Input: part model. Units: mm. Frame: model coordinates. Give positions to 0.01 mm unless a question says otherwise; leave off trailing zeros. Write each loop counter-clockwise with the first axis right and the second up, starting at its lowest first coordinate (ties: lowest second). Pieces come first, ordered by that corner, then holes. Notation, with made-up numbers: (-19.75, 66) - (-10.75, 66) arc R19 ccw to (-10.75, 90) - close; hole circle Ø7 at (-7.75, 45). An arc over 180 degrees is marked (long way). Use a Markdown table: item, result. Add a question column.
1. Section query A-A, the plane x = 113.5. Return loops of the section in (y, z).
2. Material intervals for probe 1 along Z at (x, y) = (45, -2.15); probe 2 along X at (y, z) = (-1.7, -7.5); probe 3 along X at (y, z) = (-0.35, 34), sorted ascending.
3. Section query B-B, the plane z = 38. Return loops of the section in (x, y), plus the area to 3 significant figures.
4. Pin query (flat end, axial travel): pin 1 (1.5 mm diameter, centred on x = 30.5, y = -1.5, fed in from -Z). Return the tip coordinate at first contact, or that it passes through.
5. Section query D-D, the plane z = -25. Return loops of the section in (x, y), plus the area to 3 significant figures.
6. Section query C-C, the plane y = -1.55. Count the separate pieces of the cut face and the enclosed holes in it, plus the area to 3 significant figures.
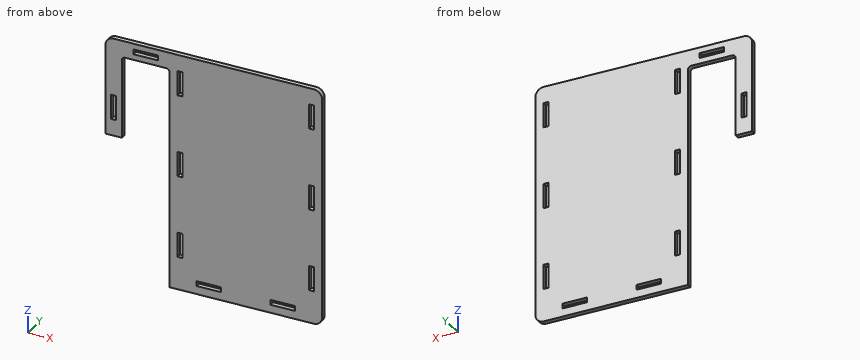
```python
from build123d import *

# Parameters (mm, degrees)
F1_W     = 15
F1_H     = 3
F1_W_2   = 3
F1_H_2   = 15
F2_DEPTH = 3


with BuildPart() as f2:
    # F1 (on Front) → F2 (new body)
    with BuildSketch(Plane.XZ):
        with BuildLine():
            Line((0, 55), (0, 0))
            Line((0, 0), (10, 0))
            Line((10, 0), (10, 48))
            ThreePointArc((10, 48), (10.5857864376, 49.4142135624), (12, 50))
            Line((12, 50), (37, 50))
            ThreePointArc((37, 50), (38.4142135624, 49.4142135624), (39, 48))
            Line((39, 48), (39, -85))
            Line((39, -85), (127, -85))
            ThreePointArc((127, -85), (130.5355339059, -83.5355339059), (132, -80))
            Line((132, -80), (132, 55))
            ThreePointArc((132, 55), (130.5355339059, 58.5355339059), (127, 60))
            Line((127, 60), (5, 60))
            ThreePointArc((5, 60), (1.4644660941, 58.5355339059), (0, 55))
        make_face()
        with Locations((63, -78.5)):
            Rectangle(F1_W, F1_H, mode=Mode.SUBTRACT)
        with Locations((45.5, -57.5)):
            Rectangle(F1_W_2, F1_H_2, mode=Mode.SUBTRACT)
        with Locations((108, -78.5)):
            Rectangle(F1_W, F1_H, mode=Mode.SUBTRACT)
        with Locations((125.5, -57.5)):
            Rectangle(F1_W_2, F1_H_2, mode=Mode.SUBTRACT)
        with Locations((5, 17.5)):
            Rectangle(F1_W_2, F1_H_2, mode=Mode.SUBTRACT)
        with Locations((45.5, -7.5)):
            Rectangle(F1_W_2, F1_H_2, mode=Mode.SUBTRACT)
        with Locations((24.5, 55)):
            Rectangle(F1_W, F1_H, mode=Mode.SUBTRACT)
        with Locations((45.5, 42.5)):
            Rectangle(F1_W_2, F1_H_2, mode=Mode.SUBTRACT)
        with Locations((125.5, -7.5)):
            Rectangle(F1_W_2, F1_H_2, mode=Mode.SUBTRACT)
        with Locations((125.5, 42.5)):
            Rectangle(F1_W_2, F1_H_2, mode=Mode.SUBTRACT)
    extrude(amount=F2_DEPTH)


solid = f2.part
```
Result sheet:
| question | item | result |
|---|---|---|
| 1 | outline | (-3, -85) - (0, -85) - (0, -80) - (-3, -80) - close; (-3, -77) - (0, -77) - (0, 60) - (-3, 60) - close |
| 2 | probe 1 | z = -85 to -65, -50 to -15, 0 to 35, 50 to 60 |
| 2 | probe 2 | x = 39 to 44, 47 to 124, 127 to 132 |
| 2 | probe 3 | x = 0 to 10, 39 to 132 |
| 3 | outline | (0, -3) - (10, -3) - (10, 0) - (0, 0) - close; (39, -3) - (44, -3) - (44, 0) - (39, 0) - close; (47, -3) - (124, -3) - (124, 0) - (47, 0) - close; (127, -3) - (132, -3) - (132, 0) - (127, 0) - close |
| 3 | area | 291 mm² |
| 4 | pin 1 | stops at z = 50 |
| 5 | outline | (39, -3) - (132, -3) - (132, 0) - (39, 0) - close |
| 5 | area | 279 mm² |
| 6 | separate pieces | 1 |
| 6 | enclosed holes | 10 |
| 6 | area | 13,900 mm² |
